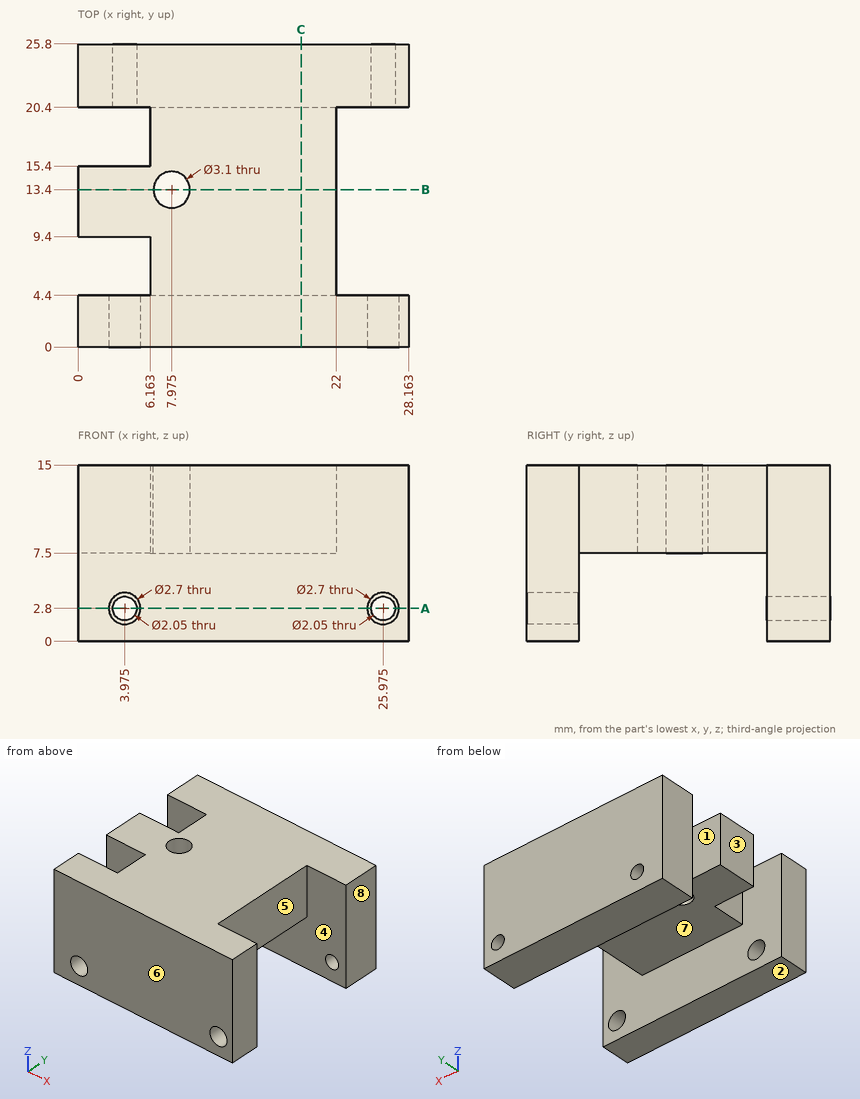
Source: three-view drawing plus pictorial views. Frame: mm from the lowest corner of the part. A direction names the side the tool comes from. Coordinates: 2 decimals unless noted, no trailing zeros. Order: outer loops, then holes, each group sorted by start corner. A loop starts at its lowest first (then second) coordinate and runs counter-clockwise, first axis right, second up.
1) Section C-C (x = 19). Return loops of the section in (y, z), then the cut area to 3 significant figures.
Result sheet:
outline: (0, 0) - (4.4, 0) - (4.4, 7.5) - (20.4, 7.5) - (20.4, 0) - (25.8, 0) - (25.8, 15) - (0, 15) - close
area: 267 mm2
2) Set-up query: the marked faces 1, 2, 3, 4 and 5. Return all of +Z, -Z, +X, -X, +Y, -Y with unobstructed straight access to the full face (end or side cutting, diameter ignored); none if empty.
Result sheet:
face 1: +Z, -Z, -X
face 2: -Z, +X, -X, +Y, -Y
face 3: +Z, -Z, -X, +Y, -Y
face 4: -Z
face 5: +Z, -Z, +X
3) First-contact query: P1, Ø3, axis at x = 6.5, y = 12, coming from the -Z side; P2, Ø2.5, axis at x = 25.975, z = 2.8, coming from the -Y side; P3, Ø6, axis at y = 11, z = 11.5, coming from the +X side. Flat tips, straight axial feed; report the tip coordinate or a pass-through.
Result sheet:
P1: stops at z = 7.5
P2: stops at y = 20.4
P3: stops at x = 22
4) Draft query along Y for the marked faces 6, 7 and 8. Return one class per face: released by +Y, released by -Y, zero draft, split by the parting line, or undercut.
Result sheet:
face 6: released by -Y
face 7: undercut
face 8: zero draft
5) Section A-A (z = 2.8). Give the number of separate pieces and of enclosed holes in the cut face, then the cut area to 3 significant figures.
Result sheet:
separate pieces: 6
enclosed holes: 0
area: 230 mm2
6) Ray query, probe 1 along X at (y, z) = (22.8, 2.8); probe 2 along Y at (x, z) = (3.75, 8.5); probe 3 along X at (y, z) = (3, 2.75). Return the intervals inside material, ascending.
Result sheet:
probe 1: x = 0 to 2.95, 5 to 24.95, 27 to 28.16
probe 2: y = 0 to 4.4, 9.4 to 15.4, 20.4 to 25.8
probe 3: x = 0 to 2.63, 5.32 to 24.63, 27.32 to 28.16
7) Section B-B (y = 13.4). Return loops of the section in (x, z) (1 decimal), then the cut area to 3 significant figures.
Result sheet:
outline: (0, 7.5) - (6.4, 7.5) - (6.4, 15) - (0, 15) - close; (9.5, 7.5) - (22, 7.5) - (22, 15) - (9.5, 15) - close
area: 142 mm2
